from build123d import *

# Parameters (mm, degrees)
SKETCH_1_W                  = 7.5
SKETCH_1_H                  = 7.5
EXTRUDE_1_DEPTH             = 40
FILLET_1_R                  = 2
HOLE_WIZARD_M2_5_1_D        = 2.05
HOLE_WIZARD_M4_1_AT_2_COUNT = 2
HOLE_WIZARD_M4_1_AT_2_PITCH = 22.5
HOLE_WIZARD_M4_1_AT_3_COUNT = 2
HOLE_WIZARD_M4_1_AT_3_PITCH = 57.118298294
HOLE_WIZARD_M4_1_AT_4_COUNT = 2
HOLE_WIZARD_M4_1_AT_4_PITCH = 52.5
FILLET_2_R                  = 2


with BuildPart() as part:
    # 草图1 → 凸台-拉伸1 (new body)
    with BuildSketch(Plane.XY):
        Polygon((7.5, 22.5), (4.5, 22.5), (4.5, 27), (-4.5, 27), (-4.5, 22.5), (-7.5, 22.5), (-7.5, 30), (7.5, 30), align=None)
        with Locations((-11.25, 26.25)):
            Rectangle(SKETCH_1_W, SKETCH_1_H)
        with Locations((11.25, 26.25)):
            Rectangle(SKETCH_1_W, SKETCH_1_H)
        Polygon((12, 22.5), (12, 19.5), (12, -19.5), (12, -22.5), (15, -22.5), (15, 22.5), align=None)
        Polygon((-12, 22.5), (-15, 22.5), (-15, -22.5), (-12, -22.5), (-12, -19.5), (-12, 19.5), align=None)
        with Locations((-11.25, -26.25)):
            Rectangle(SKETCH_1_W, SKETCH_1_H)
        with Locations((11.25, -26.25)):
            Rectangle(SKETCH_1_W, SKETCH_1_H)
        Polygon((7.5, -30), (-7.5, -30), (-7.5, -22.5), (-4.5, -22.5), (-4.5, -27), (4.5, -27), (4.5, -22.5), (7.5, -22.5), align=None)
    extrude(amount=EXTRUDE_1_DEPTH)

    # 圆角1
    fillet_1_edges = [part.edges().sort_by_distance(p)[0] for p in [
        (12, -22.5, 20),
        (12, 22.5, 20),
        (4.5, 22.5, 20),
        (4.5, 27, 20),
        (-4.5, 27, 20),
        (-4.5, 22.5, 20),
        (-12, 22.5, 20),
        (-12, -22.5, 20),
        (-4.5, -22.5, 20),
        (-4.5, -27, 20),
        (4.5, -27, 20),
        (4.5, -22.5, 20),
    ]]
    fillet(fillet_1_edges, radius=FILLET_1_R)

    # M2.5 螺纹孔1 (through all)
    with Locations(Plane(origin=(0, 30, 0), x_dir=(1, 0, 0), z_dir=(0, 1, 0))):
        with Locations((0, -38)):
            Hole(HOLE_WIZARD_M2_5_1_D / 2)

    # 草图14 → M4 螺纹孔1 (revolve, cut)
    with BuildSketch(Plane(origin=(11.25, 26.25, 0), x_dir=(0, 1, 0), z_dir=(1, 0, 0))):
        Polygon((0, 0), (0, 8.991420021), (1.65, 8), (1.65, 0), align=None)
    hole_wizard_m4_1 = revolve(axis=Axis((11.25, 26.25, -6.35), (0, 0, 1)), mode=Mode.SUBTRACT)

    # M4 螺纹孔1 at 2: M4 螺纹孔1 ×2
    with Locations(*[(-i * HOLE_WIZARD_M4_1_AT_2_PITCH, 0, 0) for i in range(1, HOLE_WIZARD_M4_1_AT_2_COUNT)]):
        add(hole_wizard_m4_1, mode=Mode.SUBTRACT)

    # M4 螺纹孔1 at 3: M4 螺纹孔1 ×2
    with Locations(*[Vector(-0.393919299, -0.91914503, 0) * (i * HOLE_WIZARD_M4_1_AT_3_PITCH) for i in range(1, HOLE_WIZARD_M4_1_AT_3_COUNT)]):
        add(hole_wizard_m4_1, mode=Mode.SUBTRACT)

    # M4 螺纹孔1 at 4: M4 螺纹孔1 ×2
    with Locations(*[(0, -i * HOLE_WIZARD_M4_1_AT_4_PITCH, 0) for i in range(1, HOLE_WIZARD_M4_1_AT_4_COUNT)]):
        add(hole_wizard_m4_1, mode=Mode.SUBTRACT)

    # 镜向1: M4 螺纹孔1 across plane
    add(hole_wizard_m4_1.mirror(Plane(origin=(0, 0, 20), x_dir=(1, 0, 0), z_dir=(0, 0, -1))), mode=Mode.SUBTRACT)

    # 镜向1 copy 1 sketch → 镜向1 copy 1 (revolve, cut)
    with BuildSketch(Plane(origin=(-11.25, 26.25, 40), x_dir=(0, 1, 0), z_dir=(1, 0, 0))):
        Polygon((0, 0), (0, -8.991420021), (1.65, -8), (1.65, 0), align=None)
    revolve(axis=Axis((-11.25, 26.25, 46.35), (0, 0, 1)), mode=Mode.SUBTRACT)

    # 镜向1 copy 2 sketch → 镜向1 copy 2 (revolve, cut)
    with BuildSketch(Plane(origin=(-11.25, -26.25, 40), x_dir=(0, 1, 0), z_dir=(1, 0, 0))):
        Polygon((0, 0), (0, -8.991420021), (1.65, -8), (1.65, 0), align=None)
    revolve(axis=Axis((-11.25, -26.25, 46.35), (0, 0, 1)), mode=Mode.SUBTRACT)

    # 镜向1 copy 3 sketch → 镜向1 copy 3 (revolve, cut)
    with BuildSketch(Plane(origin=(11.25, -26.25, 40), x_dir=(0, 1, 0), z_dir=(1, 0, 0))):
        Polygon((0, 0), (0, -8.991420021), (1.65, -8), (1.65, 0), align=None)
    revolve(axis=Axis((11.25, -26.25, 46.35), (0, 0, 1)), mode=Mode.SUBTRACT)

    # 圆角2
    fillet_2_edges = [part.edges().sort_by_distance(p)[0] for p in [
        (-15, -30, 20),
        (-15, 30, 20),
        (15, 30, 20),
        (15, -30, 20),
    ]]
    fillet(fillet_2_edges, radius=FILLET_2_R)


solid = part.part
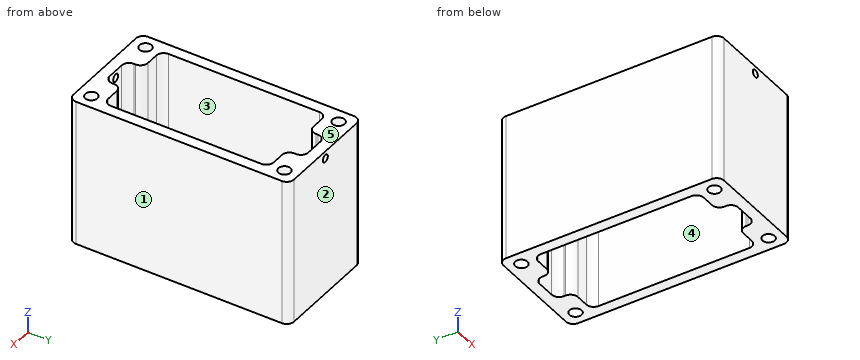
Input: part model. Units: mm. Frame: model coordinates. Face numbers are marked on the shaded views. A direction names the side the tool comes from. Round coordinates to 2 decimals unless told otherwise and drop trailing zeros. Order: outer loops, then holes, each group sorted by start corner. A loop starts at its lowest first (then second) coordinate and runs counter-clockwise, first axis right, second up. Notation, with made-up numbers: (-35, 11.25) - (6, 11.25) arc R22 ccw to (6, 35.25) - close; hole circle Ø7 at (79.5, 44.25). An arc over 180 degrees is marked (long way). Answer as a JSON object with one key per item and string values. Group by question number.
(1) Draft query along X for the marked faces 1, 2 and 3. Return one class per face: released by +X, released by -X, zero draft, split by the parting line, or undercut.
(2) Pin query (flat end, axial travel): P1, Ø3, axis at x = 11.25, y = -26.25, coming from the +Z side; P2, Ø1.8, axis at x = 0, z = 38, coming from the -Y side. Return the tip coordinate at first contact, or that it passes through.
(3) Reachability of the marked faces 4 and 5 from +Z, -Z, +X, -X, +Y, -Y: full face, straight path, thin tool, end or side. Return the list, or none.
(4) Cut plane B-B (z = 38). Count the separate pieces of the cut face and the enclosed holes in it, then the cut area to 3 significant figures.
(5) Material intervals for probe 1 along X at (y, z) = (19, 14.5); probe 2 along X at (y, z) = (-26.25, 35.75); probe 3 along Z at (x, y) = (0, -29.15) (3 decimals), sorted ascending. Write a range as from..to.
(6) Cut plane A-A (x = 0). Return loops of the section in (y, z) (3 decimals), then the cut area to 3 significant figures.
(7) Cut plane C-C (x = 7.25). Return loops of the section in (y, z), then the cut area to 3 significant figures.
Here are the results:
{
 "1": {"face 1": "released by +X", "face 2": "zero draft", "face 3": "undercut"},
 "2": {"P1": "stops at z = 31.91", "P2": "passes through"},
 "3": {"face 4": "+Z, -Z", "face 5": "+Z, +X, -X, +Y, -Y"},
 "4": {"separate pieces": "2", "enclosed holes": "4", "area": "592 mm^2"},
 "5": {"probe 1": "x = -15..-12, 12..15", "probe 2": "x = -15..-12.9, -9.6..-4.06, 4.06..9.6, 12.9..15", "probe 3": "z = 0..36.975, 39.025..40"},
 "6": {"outline": "(-30, 0) - (-27, 0) - (-27, 36.975) - (-30, 36.975) - close; (-30, 39.025) - (-27, 39.025) - (-27, 40) - (-30, 40) - close; (27, 0) - (30, 0) - (30, 36.975) - (27, 36.975) - close; (27, 39.025) - (30, 39.025) - (30, 40) - (27, 40) - close", "area": "228 mm^2"},
 "7": {"outline": "(-30, 0) - (-22.5, 0) - (-22.5, 40) - (-30, 40) - close; (22.5, 0) - (30, 0) - (30, 40) - (22.5, 40) - close", "area": "600 mm^2"}
}
